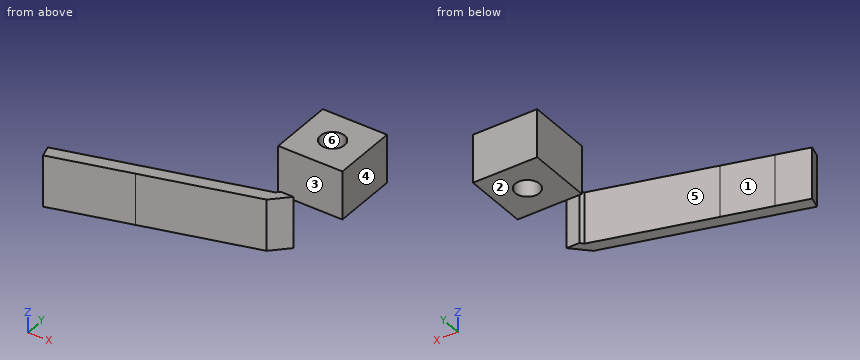
from build123d import *

# Parameters (mm, degrees)
CROQUIS1_W              = 40
CROQUIS1_H              = 40
SALIENTE_EXTRUIR1_DEPTH = 30
CROQUIS2_R              = 7.5
CORTAR_EXTRUIR1_DEPTH   = 30
SALIENTE_EXTRUIR2_DEPTH = 60
CORTAR_EXTRUIR2_DEPTH   = 28
CROQUIS5_W              = 30
CROQUIS5_H              = 32
SALIENTE_EXTRUIR3_DEPTH = 7.555544
CROQUIS6_W              = 20
CROQUIS6_H              = 32
SALIENTE_EXTRUIR4_DEPTH = 7.555546


with BuildPart() as part:
    # Croquis1 → Saliente-Extruir1 (new body)
    with BuildSketch(Plane.XY):
        with Locations((20, 20)):
            Rectangle(CROQUIS1_W, CROQUIS1_H)
    extrude(amount=SALIENTE_EXTRUIR1_DEPTH)

    # Croquis2 → Cortar-Extruir1 (cut)
    with BuildSketch(Plane.XY.offset(30)):
        with Locations((20, 20)):
            Circle(CROQUIS2_R)
    extrude(amount=-CORTAR_EXTRUIR1_DEPTH, mode=Mode.SUBTRACT)

    # Croquis3 → Saliente-Extruir2 (add)
    with BuildSketch(Plane.XY.offset(30)):
        Polygon((1.49506347, 0), (9.49506347, 0), (-0.374188302, -9.869251771), (-68.777675608, -29.117470727), (-70.824265709, -21.844387418), (-0.374188302, -2.020273637), align=None)
    extrude(amount=-SALIENTE_EXTRUIR2_DEPTH)

    # Croquis4 → Cortar-Extruir2 (cut)
    with BuildSketch(Plane.XY.offset(30)):
        Polygon((-70.824265709, -21.844387418), (-68.777675608, -29.117470727), (-0.374188302, -9.869251771), (9.49506347, 0), (1.49506347, 0), (-0.374188302, -2.020273637), align=None)
    extrude(amount=-CORTAR_EXTRUIR2_DEPTH, mode=Mode.SUBTRACT)

    # Croquis5 → Saliente-Extruir3 (add)
    with BuildSketch(Plane(origin=(2.545913561, -9.047557407, 0), x_dir=(0.9626152142655234, 0.2708725701589966, 0), z_dir=(0.2708725701589965, -0.9626152142655233, 0))):
        with Locations((-89.093561074, -14)):
            Rectangle(CROQUIS5_W, CROQUIS5_H)
    extrude(amount=-SALIENTE_EXTRUIR3_DEPTH)

    # Croquis6 → Saliente-Extruir4 (add)
    with BuildSketch(Plane(origin=(2.545913561, -9.047557407, 0), x_dir=(0.9626152142655234, 0.2708725701589966, 0), z_dir=(0.2708725701589965, -0.9626152142655233, 0))):
        with Locations((-114.093561074, -14)):
            Rectangle(CROQUIS6_W, CROQUIS6_H)
    extrude(amount=-SALIENTE_EXTRUIR4_DEPTH)


solid = part.part
Here's how the part is built. I have some questions about the finished solid (model axes, mm). Face numbers are marked on the shaded views. A direction names the side the tool comes from. Round coordinates to 2 decimals unless told otherwise and drop trailing zeros. Write each loop counter-clockwise with the first axis right and the second up, starting at its lowest first coordinate (ties: lowest second). Pieces come first, ordered by that corner, then holes. Notation, with made-up numbers: (74, 72.25) -> (85, 72.25) arc R31 ccw to (85, 104.25) -> close; hole circle Ø1 at (-26, -31.75). An arc over 180 degrees is marked (long way). One line per item, written item: value.
1) We'd pull the mould along X, two halves only. Please class the marked faces 3, 4, 5 and 6: released by +X, released by -X, zero draft, split by the parting line, or undercut.
Filled sheet:
face 3: zero draft
face 4: released by +X
face 5: released by -X
face 6: undercut
2) Suppose I cut it at A-A on y = 20. List the corners of the cut face in (x, z) for me, plus the area to 3 significant figures.
Filled sheet:
outline: (0, 0) -> (12.5, 0) -> (12.5, 30) -> (0, 30) -> close; (27.5, 0) -> (40, 0) -> (40, 30) -> (27.5, 30) -> close
area: 750 mm2
3) If I drill on line 1 (Y direction, x = 20, z = 19.5); line 2 (X direction, y = 6.5, z = 22.5); line 3 (Z direction, x = -44, y = -16), over which ranges is the centre line in solid material (lowest first)? Write a range as [from, to].
Filled sheet:
line 1: y = [0, 12.5], [27.5, 40]
line 2: x = [0, 40]
line 3: z = [-30, 2]
4) Suppose I cut it at D-D on z = 10. List the corners of the cut face in (x, y) for me.
Filled sheet:
outline: (0, 0) -> (40, 0) -> (40, 40) -> (0, 40) -> close; hole circle Ø15 at (20, 20)
5) I'm going to push flat-ended pins straight in: pin 1 Ø9 at (y, z) = (11.5, 12.5) entering from -X; pin 2 Ø9 at (x, z) = (3.5, -19) entering from +Y; pin 3 Ø3 at (x, z) = (-89.5, 2) entering from +Y. Where does each tip first touch, or does it pass through?
Filled sheet:
pin 1: stops at x = 0
pin 2: stops at y = 0
pin 3: stops at y = -26.68
6) For the marked faces 1 and 2, which set-ups out of +Z, -Z, +X, -X, +Y, -Y let a thin tool reach every point of the face, with its end or its side?
Filled sheet:
face 1: +Z, -Z, -X, +Y
face 2: -Z, +X, -X, +Y
